The listing builds one solid part. Answer for the finished solid, in the listing's coordinates (mm). A direction names the side the tool comes from. Round coordinates to 2 decimals unless told otherwise and drop trailing zeros. Write each loop counter-clockwise with the first axis right and the second up, starting at its lowest first coordinate (ties: lowest second). Pieces come first, ordered by that corner, then holes.
(1) For faces 1 (the face through (15.815, 0.986, 6.141)), 2 (the face through (15.61, 0.99, -6.04)), 3 (the face through (21.865, 0.986, 4.877)), determine the directions among +Z, -Z, +X, -X, +Y, -Y from which every point of the face is accessible in a straight line to the end or side of a thin tool.
(2) Find the intervals of material crossed by probe 1 along X at (y, z) = (1.1, 5); probe 2 along X at (y, z) = (0.4, -1.75); probe 3 along X at (y, z) = (0.9, 4.25), in increasing order.
(3) The mould has two halves that part along Z. Classify faces 4 (the face through (9, 1, 4.68)), 5 (the face through (21.61, 0.99, -5.18)), 6 (the face through (9, 0, 0)), 7 (the face through (9, 1, -4.388)): +Z half, -Z half, draft (parallel to the pull), parting line (faces both ways), or undercut.
(4) A cutting plane is placed at A-A, the plane x = 20.6. Give the vertices of the cut face in (y, z).
(5) A cutting plane is placed at B-B, the plane x = 0. Give the vertices of the cut face in (y, z).
(6) A cutting plane is placed at C-C, the plane y = 0.4. Give the vertices of the cut face in (x, z).
(7) A cutting plane is placed at D-D, the plane z = -6.5. Give the vertices of the cut face in (x, y).
(8) Each of these flat-tipped pins is pushed along its axis until it touches: pin 1 Ø1 at (x, y) = (9, 1) entering from -Z; pin 2 Ø1.5 at (x, z) = (13.5, -4) entering from -Y. Where does it stop, or does it pass through?
from build123d import *

# Parameters (mm, degrees)
SKETCH1_R           = 7
BOSS_EXTRUDE1_DEPTH = 2
SKETCH2_R           = 3.75
CUT_EXTRUDE1_DEPTH  = 11.099504938
BOSS_EXTRUDE2_START = -2
SKETCH3_R           = 1.5
BOSS_EXTRUDE2_DEPTH = 2


with BuildPart() as part:
    # Sketch1 → Boss-Extrude1 (new body)
    with BuildSketch(Plane(origin=(0, 0, 0), x_dir=(1, 0, 0), z_dir=(0, 1, 0))):
        with Locations(Location((0, 0, 0), (0, 0, 270))):
            Circle(SKETCH1_R)
    extrude(amount=BOSS_EXTRUDE1_DEPTH)

    # Sketch2 → Cut-Extrude1 (cut, through all)
    with BuildSketch(Plane(origin=(0, 2, 0), x_dir=(1, 0, 0), z_dir=(0, 1, 0))):
        with Locations(Location((0, 0, 0), (0, 0, 270))):
            Circle(SKETCH2_R)
    extrude(amount=-CUT_EXTRUDE1_DEPTH, mode=Mode.SUBTRACT)

    # Sketch3 → Boss-Extrude2 (add)
    with BuildSketch(Plane(origin=(0, 2, 0), x_dir=(1, 0, 0), z_dir=(0, 1, 0)).offset(BOSS_EXTRUDE2_START)):
        with BuildLine():
            Line((18.802724006, 7.643943352), (12.328977552, 4.387988089))
            Line((12.328977552, 4.387988089), (5.453949077, 4.387988089))
            ThreePointArc((5.453949077, 4.387988089), (6.602183106, 2.326193937), (7, 0))
            ThreePointArc((7, 0), (6.535978508, -2.506189327), (5.205432874, -4.680114165))
            Line((5.205432874, -4.680114165), (12.909805603, -4.680114165))
            Line((12.909805603, -4.680114165), (18.802724006, -7.643943352))
            ThreePointArc((18.802724006, -7.643943352), (24.183733746, -5.847211141), (22.356172256, -0.476593721))
            Line((22.356172256, -0.476593721), (21.164441, 0))
            Line((21.164441, 0), (22.356172256, 0.476593721))
            ThreePointArc((22.356172256, 0.476593721), (24.183733746, 5.847211141), (18.802724006, 7.643943352))
        make_face()
        with Locations(Location((20.6, -4.070457799, 0), (0, 0, 270))):
            Circle(SKETCH3_R, mode=Mode.SUBTRACT)
        with Locations(Location((20.6, 4.070457799, 0), (0, 0, 270))):
            Circle(SKETCH3_R, mode=Mode.SUBTRACT)
    extrude(amount=BOSS_EXTRUDE2_DEPTH)


solid = part.part
Solutions:
1. face 1: +Z, +Y, -Y
1. face 2: -Z, +Y, -Y
1. face 3: +Y, -Y
2. probe 1: x = -4.9 to 4.9, 13.55 to 19.42, 21.78 to 24.49
2. probe 2: x = -6.78 to -3.32, 3.32 to 23.86
2. probe 3: x = -5.56 to 19.11, 22.09 to 24.6
3. face 4: +Z half
3. face 5: undercut
3. face 6: draft
3. face 7: -Z half
4. outline: (0, -8.07) - (2, -8.07) - (2, -5.57) - (0, -5.57) - close; (0, -2.57) - (2, -2.57) - (2, 2.57) - (0, 2.57) - close; (0, 5.57) - (2, 5.57) - (2, 8.07) - (0, 8.07) - close
5. outline: (0, -7) - (2, -7) - (2, -3.75) - (0, -3.75) - close; (0, 3.75) - (2, 3.75) - (2, 7) - (0, 7) - close
6. outline: (5.21, 4.68) arc R7 ccw (long way) to (5.45, -4.39) - (12.33, -4.39) - (18.8, -7.64) arc R4 ccw (long way) to (22.36, -0.48) - (21.16, 0) - (22.36, 0.48) arc R4 ccw (long way) to (18.8, 7.64) - (12.91, 4.68) - close; hole circle Ø7.5 at (0, 0); hole circle Ø3 at (20.6, -4.07); hole circle Ø3 at (20.6, 4.07)
7. outline: (-2.6, 0) - (2.6, 0) - (2.6, 2) - (-2.6, 2) - close; (16.53, 0) - (23.78, 0) - (23.78, 2) - (16.53, 2) - close
8. pin 1: stops at z = -4.39
8. pin 2: stops at y = 0
